CAD build for the part. Positions are in the model's coordinates, mm. A direction names the side the tool comes from. Round coordinates to 2 decimals unless told otherwise and drop trailing zeros. Order: outer loops, then holes, each group sorted by start corner. A loop starts at its lowest first (then second) coordinate and runs counter-clockwise, first axis right, second up.
```python
from build123d import *

# Parameters (mm, degrees)
F1_DEPTH = 50.8
F0_W     = 76.2
F0_H     = 25.4
F2_DEPTH = 25.4


with BuildPart() as f1:
    # F0 (on Top) → F1 (new body)
    with BuildSketch(Plane.XY):
        Polygon((7.2523672134, 33.3039297216), (-68.9476327866, 33.3039297216), (-68.9476327866, -42.8960702784), (7.2523672134, -42.8960702784), (7.2523672134, -17.4960702784), (83.4523672134, -17.4960702784), (83.4523672134, 7.9039297216), (7.2523672134, 7.9039297216), align=None)
    extrude(amount=F1_DEPTH)

    # F0 (on Top) → F2 (join)
    with BuildSketch(Plane.XY):
        Polygon((7.2523672134, 33.3039297216), (-68.9476327866, 33.3039297216), (-68.9476327866, -42.8960702784), (7.2523672134, -42.8960702784), (7.2523672134, -17.4960702784), (83.4523672134, -17.4960702784), (83.4523672134, 7.9039297216), (7.2523672134, 7.9039297216), align=None)
        with Locations((45.3523672134, 20.6039297216)):
            Rectangle(F0_W, F0_H)
        with Locations((45.3523672134, -30.1960702784)):
            Rectangle(F0_W, F0_H)
    extrude(amount=F2_DEPTH)


solid = f1.part
```
1. Tool access for faces 1 (the face through (45, 21, 25.4)), 2 (the face through (-11, -4, 50.8)), 3 (the face through (7.252, -30, 38)): list every direction of +Z, -Z, +X, -X, +Y, -Y with a clear straight run to the whole face (end or side of a thin tool).
2. Drill centre lines: line 1 (Z direction, x = 17, y = -39); line 2 (X direction, y = -32, z = 34); line 3 (Y direction, x = 33, z = 48.5). Where is each one in solid material? Low to high.
3. Pin check, flat tips, straight feed: P1, Ø12.5, axis at x = 37, z = 42, coming from the +Y side; P2, Ø6, axis at y = 21.5, z = 39.5, coming from the +X side; P3, Ø4, axis at x = 65.5, y = -22.5, coming from the -Z side; P4, Ø12, axis at x = 48.5, z = 38, coming from the -Y side. Stop position of each tip, or through.
4. Cut at A-A, the plane x = 44. Write the cut outline in (y, z).
5. Cut at C-C, the plane y = 18.5. Write the cut outline in (x, z), and give its area (3 significant figures).
6. Cut at B-B, the plane z = 37. Write the cut outline in (x, y), and give its area (3 significant figures).
Outcome:
1. face 1: +Z, +X, +Y
1. face 2: +Z, +X, -X, +Y, -Y
1. face 3: +Z, +X, -Y
2. line 1: z = 0 to 25.4
2. line 2: x = -68.95 to 7.25
2. line 3: y = -17.5 to 7.9
3. P1: stops at y = 7.9
3. P2: stops at x = 7.25
3. P3: stops at z = 0
3. P4: stops at y = -17.5
4. outline: (-42.9, 0) - (33.3, 0) - (33.3, 25.4) - (7.9, 25.4) - (7.9, 50.8) - (-17.5, 50.8) - (-17.5, 25.4) - (-42.9, 25.4) - close
5. outline: (-68.95, 0) - (83.45, 0) - (83.45, 25.4) - (7.25, 25.4) - (7.25, 50.8) - (-68.95, 50.8) - close
5. area: 5,810 mm2
6. outline: (-68.95, -42.9) - (7.25, -42.9) - (7.25, -17.5) - (83.45, -17.5) - (83.45, 7.9) - (7.25, 7.9) - (7.25, 33.3) - (-68.95, 33.3) - close
6. area: 7,740 mm2
